```python
from build123d import *

# Parameters (mm, degrees)
SKETCH1_R           = 80
SKETCH1_R_2         = 15
BOSS_EXTRUDE1_DEPTH = 20
SKETCH2_R           = 80
SKETCH2_R_2         = 75
BOSS_EXTRUDE2_DEPTH = 150
SKETCH3_R           = 95
SKETCH3_R_2         = 75
BOSS_EXTRUDE3_DEPTH = 20
FILLET1_R           = 10


with BuildPart() as part:
    # Sketch1 → Boss-Extrude1 (new body)
    with BuildSketch(Plane.XY):
        Circle(SKETCH1_R)
        Circle(SKETCH1_R_2, mode=Mode.SUBTRACT)
    extrude(amount=BOSS_EXTRUDE1_DEPTH)

    # Sketch2 → Boss-Extrude2 (add)
    with BuildSketch(Plane.XY.offset(20)):
        Circle(SKETCH2_R)
        Circle(SKETCH2_R_2, mode=Mode.SUBTRACT)
    extrude(amount=BOSS_EXTRUDE2_DEPTH)

    # Sketch3 → Boss-Extrude3 (add)
    with BuildSketch(Plane.XY.offset(170)):
        Circle(SKETCH3_R)
        Circle(SKETCH3_R_2, mode=Mode.SUBTRACT)
    extrude(amount=BOSS_EXTRUDE3_DEPTH)

    # Fillet1
    fillet1_edges = [part.edges().sort_by_distance(p)[0] for p in [
        (-80, 0, 170),
    ]]
    fillet(fillet1_edges, radius=FILLET1_R)


solid = part.part
```
Geometry check sheet. Reference: the model listing, model coordinates, mm. A direction names the side the tool comes from. Give positions to 0.01 mm unless a question says otherwise; leave off trailing zeros. Loops run counter-clockwise (first coordinate to the right, second up) from the corner with the lowest first, then second, coordinate; pieces in that order, holes last. Notation, with made-up numbers: M 63.5,-6 L 106.5,-6 A13 cw 106.5,10 Z; hole C 17.5,30 d5. An arc over 180 degrees is marked long. Write item = value, one per line.
(1) Sectioned sample at C-C, the plane z = 124.5. Record the cut outline in (x, y), plus the area to 3 significant figures.
Answer below:
outline = C 0,0 d160; hole C 0,0 d150
area = 2,430 mm2
(2) Material ranges on line 1 (Y direction, x = 0, z = 15.25); line 2 (Y direction, x = 0, z = 108); line 3 (Z direction, x = 25, y = 46), recorded low to high. Write a range as [from, to].
Answer below:
line_1 = [-80, -15], [15, 80]
line_2 = [-80, -75], [75, 80]
line_3 = [0, 20]
(3) Tool access check on faces 4 (the face through (17, 1, 0)), 5 (the face through (-57, -70, 170)), 6 (the face through (-1, -16, 20)). Record the directions out of +Z, -Z, +X, -X, +Y, -Y that give a thin tool (end or side, any length) a straight path to the whole face; none if there is none.
Answer below:
face_4 = -Z, +X, -X, +Y, -Y
face_5 = -Z
face_6 = +Z
(4) Sectioned sample at A-A, the plane y = 0. Record the cut outline in (x, z), plus the area to 3 significant figures.
Answer below:
outline = M -95,170 L -90,170 A10 cw -80,160 L -80,0 L -15,0 L -15,20 L -75,20 L -75,190 L -95,190 Z; M 15,0 L 80,0 L 80,160 A10 cw 90,170 L 95,170 L 95,190 L 75,190 L 75,20 L 15,20 Z
area = 4,940 mm2
(5) Gauge pin test, flat ends, axial feed: pin 1 Ø5 at (x, z) = (-60.5, 109) entering from +Y; pin 2 Ø10 at (x, y) = (6, 19.5) entering from +Z; pin 3 Ø10 at (y, z) = (33.5, 61.5) entering from -X. Record the tip position at first contact, or that the pin passes through.
Answer below:
pin_1 = 55.1
pin_2 = 20
pin_3 = -74.75
(6) Release check for a two-part mould opening along X. For faces 1 (the face through (-17.34, -78.1, 78.88)), 2 (the face through (70, 29, 190)), 3 (the face through (-9.764, 74.362, 103.81)) record: released by +X, released by -X, zero draft, split by the parting line, or undercut.
Answer below:
face_1 = split by the parting line
face_2 = zero draft
face_3 = undercut
